```python
from build123d import *

# Parameters (mm, degrees)
SKETCH1_W                                    = 94
SKETCH1_H                                    = 63.5
BOSS_EXTRUDE1_DEPTH                          = 4
CBORE_SLOT_FOR_M5_HEX_HEAD_BOLT1_D           = 5.8
CBORE_SLOT_FOR_M5_HEX_HEAD_BOLT1_DEPTH       = 18
CBORE_SLOT_FOR_M5_HEX_HEAD_BOLT1_CBORE_D     = 12.24
CBORE_SLOT_FOR_M5_HEX_HEAD_BOLT1_CBORE_DEPTH = 3.58
CBORE_SLOT_FOR_M5_HEX_HEAD_BOLT1_TIP         = 1.742495795
FILLET1_R                                    = 5


with BuildPart() as part:
    # Sketch1 → Boss-Extrude1 (new body)
    with BuildSketch(Plane(origin=(0, 0, 0), x_dir=(1, 0, 0), z_dir=(0, 1, 0))):
        with Locations((12.203186111, 24.532883045)):
            Rectangle(SKETCH1_W, SKETCH1_H)
    extrude(amount=BOSS_EXTRUDE1_DEPTH)

    # CBORE SLOT for M5 Hex Head Bolt1
    with Locations(Plane(origin=(0, 4, 0), x_dir=(1, 0, 0), z_dir=(0, 1, 0))):
        with Locations((-26.296813889, 47.782883045), (-26.296813889, 1.282883045), (50.753186111, 47.782883045), (50.753186111, 1.282883045), (-26.346813889, 47.782883045), (-26.346813889, 1.282883045), (50.703186111, 1.282883045), (50.703186111, 47.782883045)):
            CounterBoreHole(CBORE_SLOT_FOR_M5_HEX_HEAD_BOLT1_D / 2, CBORE_SLOT_FOR_M5_HEX_HEAD_BOLT1_CBORE_D / 2, CBORE_SLOT_FOR_M5_HEX_HEAD_BOLT1_CBORE_DEPTH, depth=CBORE_SLOT_FOR_M5_HEX_HEAD_BOLT1_DEPTH)
            with Locations((0, 0, -(CBORE_SLOT_FOR_M5_HEX_HEAD_BOLT1_DEPTH + CBORE_SLOT_FOR_M5_HEX_HEAD_BOLT1_TIP / 2))):  # 118° drill point
                Cone(0, CBORE_SLOT_FOR_M5_HEX_HEAD_BOLT1_D / 2, CBORE_SLOT_FOR_M5_HEX_HEAD_BOLT1_TIP, mode=Mode.SUBTRACT)

    # Fillet1
    fillet1_edges = [part.edges().sort_by_distance(p)[0] for p in [
        (-34.796813889, 2, -56.282883045),
        (59.203186111, 2, -56.282883045),
        (59.203186111, 2, 7.217116955),
        (-34.796813889, 2, 7.217116955),
    ]]
    fillet(fillet1_edges, radius=FILLET1_R)


solid = part.part
```
Work out the finished part from the listing and answer in its coordinate system (mm). A direction names the side the tool comes from. Give positions to 0.01 mm unless a question says otherwise; leave off trailing zeros. Order: outer loops, then holes, each group sorted by start corner. A loop starts at its lowest first (then second) coordinate and runs counter-clockwise, first axis right, second up. Notation, with made-up numbers: M -26,52 L 11,52 A23 cw 11,77 Z; hole C -25,20.5 d2. An arc over 180 degrees is marked long. Return JSON: item names as keys, results as strings.
1) A tool of negligible diameter and unlimited length cuts with its end or side. For faces 1 (the cylindrical face through (47.804, 0.207, -47.719)), 2 (the flat face through (49, 0.42, -45)), 3 (the flat face through (59.203, 2, -24)), from which of +Z, -Z, +X, -X, +Y, -Y can it reach the whole face along a straight path? Write none if from no direction.
Resolved:
{"face 1": "+Y, -Y", "face 2": "+Y", "face 3": "+Z, -Z, +X, +Y, -Y"}
2) Section B-B, the plane y = 1.75 is taken. Write down the section's boundary in (x, z), plus the area to 3 significant figures.
Resolved:
{"outline": "M -34.8,-51.28 A5 ccw -29.8,-56.28 L 54.2,-56.28 A5 ccw 59.2,-51.28 L 59.2,2.22 A5 ccw 54.2,7.22 L -29.8,7.22 A5 ccw -34.8,2.22 Z; hole M -26.32,-53.9 A6.12 ccw long -26.32,-41.66 A6.12 ccw long Z; hole M -26.32,-7.4 A6.12 ccw long -26.32,4.84 A6.12 ccw long Z; hole M 50.73,-53.9 A6.12 ccw long 50.73,-41.66 A6.12 ccw long Z; hole M 50.73,-7.4 A6.12 ccw long 50.73,4.84 A6.12 ccw long Z", "area": "5,470 mm^2"}
3) Straight lines are drawn through the part: line 1 along Z through (x, y) = (-26.5, 2.4); line 2 along Z through (x, y) = (53.5, 2.3); line 3 along X through (y, z) = (0.7, -52). For each, find the intervals that lie inside material, in ascending order. Write a range as [from, to].
Resolved:
{"line 1": "[-56.28, -53.9], [-41.66, -7.4], [4.84, 7.22]", "line 2": "[-56.28, -53.25], [-42.31, -6.75], [4.19, 7.22]", "line 3": "[-34.75, -30.78], [-21.86, 46.27], [55.19, 59.15]"}
4) Section A-A, the plane z = -1.5 is taken. Write down the section's boundary in (x, y).
Resolved:
{"outline": "M -34.8,0 L -29.24,0 L -29.24,0.42 L -32.46,0.42 L -32.46,4 L -34.8,4 Z; M -23.4,0 L 47.81,0 L 47.81,0.42 L 44.59,0.42 L 44.59,4 L -20.18,4 L -20.18,0.42 L -23.4,0.42 Z; M 53.65,0 L 59.2,0 L 59.2,4 L 56.87,4 L 56.87,0.42 L 53.65,0.42 Z"}
5) Section C-C, the plane x = -28 is taken. Write down the section's boundary in (y, z), plus the area to 3 significant figures.
Resolved:
{"outline": "M 0,-56.28 L 4,-56.28 L 4,-53.68 L 0.42,-53.68 L 0.42,-50.17 L 0,-50.17 Z; M 0,-45.4 L 0.42,-45.4 L 0.42,-41.89 L 4,-41.89 L 4,-7.18 L 0.42,-7.18 L 0.42,-3.67 L 0,-3.67 Z; M 0,1.1 L 0.42,1.1 L 0.42,4.61 L 4,4.61 L 4,7.22 L 0,7.22 Z", "area": "166 mm^2"}
6) For a pull along Z with two mould halves and no side action, classify faces 4 (the cylindrical face through (-32.465, 2.235, -47.918)), 5 (the flat face through (-27.8, 0.42, 1.4)), 6 (the flat face through (-34.797, 2, -24)), 7 (the cylindrical face through (-33.371, 2.028, 5.714)) as +Z half, -Z half, draft (parallel to the pull), parting line (faces both ways), or undercut.
Resolved:
{"face 4": "undercut", "face 5": "undercut", "face 6": "draft", "face 7": "+Z half"}
